Can you work these out from the model? Positions are in its coordinate system, mm. Face numbers are marked on the shaded views. A direction names the side the tool comes from. Coordinates: 2 decimals unless noted, no trailing zeros. Order: outer loops, then holes, each group sorted by start corner. A loop starts at its lowest first (then second) coordinate and runs counter-clockwise, first axis right, second up.
```python
from build123d import *

# Parameters (mm, degrees)
SKETCH_4_R          = 6
EXTRUDE_7_DEPTH     = 4
SKETCH_6_R          = 5.2
CUT_EXTRUDE_3_DEPTH = 3.2
EXTRUDE_8_DEPTH     = 3
EXTRUDE_9_DEPTH     = 2.2
SKETCH_8_R          = 1.5
EXTRUDE_10_DEPTH    = 3.2
EXTRUDE_11_DEPTH    = 3
SKETCH_8_8_R        = 1
EXTRUDE_12_DEPTH    = 3.8
FILLET_1_R          = 0.2


with BuildPart() as part:
    # Sketch 4 → Extrude 7 (new body)
    with BuildSketch(Plane.XY):
        Circle(SKETCH_4_R)
    extrude(amount=EXTRUDE_7_DEPTH)

    # Sketch 6 → Cut-Extrude 3 (cut)
    with BuildSketch(Plane.XY.offset(4)):
        Circle(SKETCH_6_R)
    extrude(amount=-CUT_EXTRUDE_3_DEPTH, mode=Mode.SUBTRACT)

    # Sketch 7 → Extrude 8 (add)
    with BuildSketch(Plane.XY.offset(4)):
        with BuildLine():
            Line((0.5, 6.6), (-0.5, 6.6))
            Line((-0.5, 6.6), (-0.5, 5.979130372))
            ThreePointArc((-0.5, 5.979130372), (0, 6), (0.5, 5.979130372))
            Line((0.5, 5.979130372), (0.5, 6.6))
        make_face()
        with BuildLine():
            ThreePointArc((0.75, -5.95294045), (0, -6), (-0.75, -5.95294045))
            Line((-0.75, -5.95294045), (-0.75, -6.6))
            Line((-0.75, -6.6), (0.75, -6.6))
            Line((0.75, -6.6), (0.75, -5.95294045))
        make_face()
        with BuildLine():
            ThreePointArc((-5.979130372, -0.5), (-6, 0), (-5.979130372, 0.5))
            Line((-5.979130372, 0.5), (-6.6, 0.5))
            Line((-6.6, 0.5), (-6.6, -0.5))
            Line((-6.6, -0.5), (-5.979130372, -0.5))
        make_face()
        with BuildLine():
            Line((6.6, 0.5), (5.979130372, 0.5))
            ThreePointArc((5.979130372, 0.5), (5.994780322, 0.250217676), (6, 0))
            ThreePointArc((6, 0), (5.994780322, -0.250217676), (5.979130372, -0.5))
            Line((5.979130372, -0.5), (6.6, -0.5))
            Line((6.6, -0.5), (6.6, 0.5))
        make_face()
    extrude(amount=-EXTRUDE_8_DEPTH)

    # Sketch 7_3 → Extrude 9 (add)
    with BuildSketch(Plane.XY.offset(4)):
        with BuildLine():
            Line((0.5, 6.6), (-0.5, 6.6))
            Line((-0.5, 6.6), (-0.5, 5.979130372))
            ThreePointArc((-0.5, 5.979130372), (0, 6), (0.5, 5.979130372))
            Line((0.5, 5.979130372), (0.5, 6.6))
        make_face()
        with BuildLine():
            ThreePointArc((0.5, 5.979130372), (0, 6), (-0.5, 5.979130372))
            Line((-0.5, 5.979130372), (-0.5, 5.175905718))
            ThreePointArc((-0.5, 5.175905718), (0, 5.2), (0.5, 5.175905718))
            Line((0.5, 5.175905718), (0.5, 5.979130372))
        make_face()
    extrude(amount=EXTRUDE_9_DEPTH)

    # Sketch 8 → Extrude 10 (add)
    with BuildSketch(Plane.XY.offset(0.8)):
        Circle(SKETCH_8_R)
    extrude(amount=EXTRUDE_10_DEPTH)

    # Sketch 8_3 → Extrude 11 (add)
    with BuildSketch(Plane.XY.offset(0.8)):
        with BuildLine():
            Line((-1.414213562, 0.5), (-3, 0.5))
            Line((-3, 0.5), (-3, -0.5))
            Line((-3, -0.5), (-1.414213562, -0.5))
            ThreePointArc((-1.414213562, -0.5), (-1.5, 0), (-1.414213562, 0.5))
        make_face()
        with BuildLine():
            Line((-0.5, 3), (-0.5, 1.414213562))
            ThreePointArc((-0.5, 1.414213562), (0, 1.5), (0.5, 1.414213562))
            Line((0.5, 1.414213562), (0.5, 3))
            Line((0.5, 3), (-0.5, 3))
        make_face()
        with BuildLine():
            Line((3, 0.5), (1.414213562, 0.5))
            ThreePointArc((1.414213562, 0.5), (1.478397839, 0.253652968), (1.5, 0))
            ThreePointArc((1.5, 0), (1.478397839, -0.253652968), (1.414213562, -0.5))
            Line((1.414213562, -0.5), (3, -0.5))
            Line((3, -0.5), (3, 0.5))
        make_face()
        with BuildLine():
            ThreePointArc((0.5, -1.414213562), (0, -1.5), (-0.5, -1.414213562))
            Line((-0.5, -1.414213562), (-0.5, -3))
            Line((-0.5, -3), (0.5, -3))
            Line((0.5, -3), (0.5, -1.414213562))
        make_face()
    extrude(amount=EXTRUDE_11_DEPTH)

    # Sketch 8_8 → Extrude 12 (add)
    with BuildSketch(Plane.XY.offset(0.8)):
        Circle(SKETCH_8_8_R)
    extrude(amount=EXTRUDE_12_DEPTH)

    # Fillet 1
    fillet_1_edges = [part.edges().sort_by_distance(p)[0] for p in [
        (-1, 0, 4.6),
        (0.5, 5.887952859, 6.2),
        (0, 6.6, 6.2),
        (-0.5, 5.887952859, 6.2),
        (0, 5.2, 6.2),
    ]]
    fillet(fillet_1_edges, radius=FILLET_1_R)


solid = part.part
```
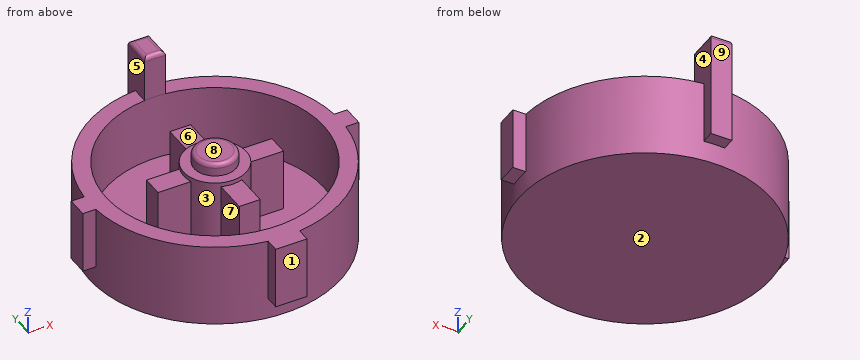
1. On a 3-axis mill with a long thin cutter (end or side, diameter ignored), from which of +Z, -Z, +X, -X, +Y, -Y can I reach the whole of each face in a straight line? I mean the marked faces 1, 2, 3, 4 and 5. Say none if no direction works.
Completed:
face 1: +Z, -Z, +X, -X, -Y
face 2: -Z, +X, -X, +Y, -Y
face 3: +Z
face 4: +Z, +X, +Y
face 5: +Z, -X, +Y
2. Imagine slicing it at B-B on x = 0. Please give me the cut outline in (y, z).
Completed:
outline: (-6.6, 1) - (-6, 1) - (-6, 0) - (6, 0) - (6, 1) - (6.6, 1) - (6.6, 6) arc R0.2 ccw to (6.4, 6.2) - (5.4, 6.2) arc R0.2 ccw to (5.2, 6) - (5.2, 0.8) - (3, 0.8) - (3, 3.8) - (1.5, 3.8) - (1.5, 4) - (1, 4) - (1, 4.4) arc R0.2 ccw to (0.8, 4.6) - (-0.8, 4.6) arc R0.2 ccw to (-1, 4.4) - (-1, 4) - (-1.5, 4) - (-1.5, 3.8) - (-3, 3.8) - (-3, 0.8) - (-5.2, 0.8) - (-5.2, 4) - (-6.6, 4) - close
3. Please list where these lines run through material, in increasing order: probe 1 along X at (y, z) = (0, 1.9); probe 2 along Y at (x, z) = (-1.75, 2.75).
Completed:
probe 1: x = -6.6 to -5.2, -3 to 3, 5.2 to 6.6
probe 2: y = -5.74 to -4.9, -0.5 to 0.5, 4.9 to 5.74
4. Imagine slicing it at C-C on y = 0. Please give me the cut outline in (x, z), then the cut area to 3 significant figures.
Completed:
outline: (-6.6, 1) - (-6, 1) - (-6, 0) - (6, 0) - (6, 1) - (6.6, 1) - (6.6, 4) - (5.2, 4) - (5.2, 0.8) - (3, 0.8) - (3, 3.8) - (1.5, 3.8) - (1.5, 4) - (1, 4) - (1, 4.4) arc R0.2 ccw to (0.8, 4.6) - (-0.8, 4.6) arc R0.2 ccw to (-1, 4.4) - (-1, 4) - (-1.5, 4) - (-1.5, 3.8) - (-3, 3.8) - (-3, 0.8) - (-5.2, 0.8) - (-5.2, 4) - (-6.6, 4) - close
area: 38.1 mm2
5. Thinking about a two-plate mould opening in Y: for the marked faces 6, 7, 8 and 9, which applies, pulls with the +Y half, pulls with the -Y half, needs draft (parallel to the pull), parting line crosses it, or undercut?
Completed:
face 6: undercut
face 7: undercut
face 8: needs draft
face 9: pulls with the +Y half
6. I'm going to push flat-ended pins straight in: pin 1 (1.3 mm diameter, centred on x = -2, z = 2.5, fed in from -Y); pin 2 (0.5 mm diameter, centred on y = -2, z = 2.5, fed in from +X); pin 3 (0.8 mm diameter, centred on y = -2.5, z = 2, fed in from -X). Where does each tip first touch, or does it pass through?
Completed:
pin 1: stops at y = -5.85
pin 2: stops at x = 5.74
pin 3: stops at x = -5.62
7. Imagine slicing it at D-D on y = -5. Please give me the cut outline in (x, z), then the cut area to 3 significant figures.
Completed:
outline: (-3.32, 0) - (3.32, 0) - (3.32, 4) - (1.43, 4) - (1.43, 0.8) - (-1.43, 0.8) - (-1.43, 4) - (-3.32, 4) - close
area: 17.4 mm2
8. Imagine slicing it at A-A on z = 2.5. Give the number of separate pieces and of enclosed holes in the cut face, then the cut area to 3 significant figures.
Completed:
separate pieces: 2
enclosed holes: 1
area: 44.1 mm2
